from build123d import *

# Parameters (mm, degrees)
BOSS_EXTRU_1_DEPTH      = 42
ESQUISSE2_R             = 2.5
ENL_V_MAT_EXTRU_1_DEPTH = 42
ESQUISSE4_R             = 3.5
ENL_V_MAT_EXTRU_2_DEPTH = 8.5
ENL_V_MAT_EXTRU_4_DEPTH = 47
BOSS_EXTRU_2_START      = -1
ESQUISSE6_R             = 3.5
ESQUISSE6_R_2           = 1.5
ESQUISSE6_R_3           = 1.6
BOSS_EXTRU_2_DEPTH      = 1


with BuildPart() as part:
    # Esquisse1 → Boss.-Extru.1 (new body)
    with BuildSketch(Plane.XY):
        Polygon((0, 3.5), (5, 3.5), (5, 0), (15, 0), (15, 8), (0, 8), align=None)
    extrude(amount=BOSS_EXTRU_1_DEPTH)

    # Esquisse2 → Enlèv. mat.-Extru.1 (cut)
    with BuildSketch(Plane(origin=(0, 8, 0), x_dir=(1, 0, 0), z_dir=(0, 1, 0))):
        with Locations(Location((9.5, -5.5, 0), (0, 0, 270))):
            Circle(ESQUISSE2_R)
        with Locations(Location((9.5, -36.5, 0), (0, 0, 270))):
            Circle(ESQUISSE2_R)
    extrude(amount=-ENL_V_MAT_EXTRU_1_DEPTH, mode=Mode.SUBTRACT)

    # Esquisse4 → Enlèv. mat.-Extru.2 (cut)
    with BuildSketch(Plane(origin=(0, 8, 0), x_dir=(1, 0, 0), z_dir=(0, 1, 0))):
        with Locations(Location((9.5, -5.5, 0), (0, 0, 270))):
            Circle(ESQUISSE4_R)
        with Locations(Location((9.5, -36.5, 0), (0, 0, 270))):
            Circle(ESQUISSE4_R)
    extrude(amount=-ENL_V_MAT_EXTRU_2_DEPTH, mode=Mode.SUBTRACT)

    # Esquisse5 → Enlèv. mat.-Extru.4 (cut)
    with BuildSketch(Plane.XY.offset(42)):
        Polygon((5, 8), (15, 3), (18.054100071, 8.962914679), (5.626380762, 14.083983342), align=None)
    extrude(amount=-ENL_V_MAT_EXTRU_4_DEPTH, mode=Mode.SUBTRACT)

    # Esquisse6 → Boss.-Extru.2 (add)
    # profile 1 of 2: a face of its own
    with BuildSketch(Plane(origin=(0, 0, 0), x_dir=(-1, 0, 0), z_dir=(0, -1, 0)).offset(BOSS_EXTRU_2_START)):
        with Locations((-9.5, -36.5)):
            Circle(ESQUISSE6_R)
        with Locations(Location((-9.5, -36.5, 0), (0, 0, 90))):
            Circle(ESQUISSE6_R_2, mode=Mode.SUBTRACT)
    # profile 2 of 2: a face of its own
    with BuildSketch(Plane(origin=(0, 0, 0), x_dir=(-1, 0, 0), z_dir=(0, -1, 0)).offset(BOSS_EXTRU_2_START)):
        with Locations((-9.5, -5.5)):
            Circle(ESQUISSE6_R)
        with Locations(Location((-9.5, -5.5, 0), (0, 0, 90))):
            Circle(ESQUISSE6_R_3, mode=Mode.SUBTRACT)
    extrude(amount=BOSS_EXTRU_2_DEPTH)


solid = part.part
Geometry: final body of the model. Coordinates: model frame, mm. A direction names the side the tool comes from. Coordinates: 2 decimals unless noted, no trailing zeros. Order: outer loops, then holes, each group sorted by start corner. A loop starts at its lowest first (then second) coordinate and runs counter-clockwise, first axis right, second up. Notation, with made-up numbers: (-7.5, 54.5) - (32.5, 54.5) arc R32 ccw to (32.5, 81.5) - close; hole circle Ø11 at (13.25, 86.5). An arc over 180 degrees is marked (long way). Use one line per item in the form item = value.
1) Set-up query: faces 1 (the face through (9.93, 5.535, 21.294)), 2 (the face through (8, 1, 37.2)), 3 (the face through (2, 3.5, 21)). Return all of +Z, -Z, +X, -X, +Y, -Y with unobstructed straight access to the full face (end or side cutting, diameter ignored); none if empty.
Solutions:
face_1 = +Z, -Z, +X, +Y
face_2 = +Y
face_3 = +Z, -Z, -X, -Y
2) Section A-A (x = 9.5). Return loops of the section in (y, z).
Solutions:
outline = (0, 0) - (5.75, 0) - (5.75, 2) - (1, 2) - (1, 3.9) - (0, 3.9) - close; (0, 7.1) - (1, 7.1) - (1, 9) - (5.75, 9) - (5.75, 33) - (1, 33) - (1, 35) - (0, 35) - close; (0, 38) - (1, 38) - (1, 40) - (5.75, 40) - (5.75, 42) - (0, 42) - close
3) Pin query (flat end, axial travel): pin 1 (5.5 mm diameter, centred on x = 9.5, z = 37, fed in from +Y); pin 2 (1 mm diameter, centred on x = 11, y = 7, fed in from -Z); pin 3 (2.5 mm diameter, centred on x = 3, z = 31, fed in from -Y); pin 4 (6 mm diameter, centred on x = 13.5, z = 30.5, fed in from +Y). Return the tip coordinate at first contact, or that it passes through.
Solutions:
pin_1 = 1
pin_2 = through
pin_3 = 3.5
pin_4 = 5.25
4) Section B-B (z = 5.5). Return loops of the section in (x, y), then the cut area to 4 significant figures.
Solutions:
outline = (0, 3.5) - (5, 3.5) - (5, 0) - (7.9, 0) - (7.9, 1) - (6, 1) - (6, 7.5) - (5, 8) - (0, 8) - close; (11.1, 0) - (15, 0) - (15, 3) - (13, 4) - (13, 1) - (11.1, 1) - close
area = 41.05 mm^2
5) Section D-D (z = 16). Return loops of the section in (x, y).
Solutions:
outline = (0, 3.5) - (5, 3.5) - (5, 0) - (15, 0) - (15, 3) - (5, 8) - (0, 8) - close
6) Mould query, pull axis Z, two halves, no side actions, for faces 4 (the face through (6.083, 3.573, 35.741)), 5 (the face through (7, 4, 0)), 6 (the face through (5, 2, 21)), 7 (the face through (6.083, 3.573, 4.741)). Classes: +Z half, -Z half, draft (parallel to the pull), parting line (faces both ways), or undercut.
Solutions:
face_4 = undercut
face_5 = -Z half
face_6 = draft
face_7 = undercut
7) Section C-C (y = 0.5). Return loops of the section in (x, z), then the cut area to 3 significant figures.
Solutions:
outline = (5, 0) - (15, 0) - (15, 42) - (5, 42) - close; hole circle Ø3.2 at (9.5, 5.5); hole circle Ø3 at (9.5, 36.5)
area = 405 mm^2
8) Ray query, L1, parallel to Z at x = 9.75, y = 2.5; L2, parallel to Y at x = 2.25, z = 17.5; L3, parallel to X at y = 5, z = 5.5. Return the intervals inside material, ascending.
Solutions:
L1 = 0 to 2.01, 8.99 to 33.01, 39.99 to 42
L2 = 3.5 to 8
L3 = 0 to 6
